Verification items for this drawing (mm, ordinates from the low corner). Give positions to 0.01 mm unless a question says otherwise; leave off trailing zeros. Write each loop counter-clockwise with the first axis right and the second up, starting at its lowest first coordinate (ties: lowest second). Pieces come first, ordered by that corner, then holes. Notation, with made-up numbers: (64.5, -33.75) -> (69.5, -33.75) arc R16 ccw to (69.5, -13.75) -> close; hole circle Ø7 at (13.5, -0.5). An arc over 180 degrees is marked (long way). Use one line per item in the form item = value. Start each with the question number.
(1) Depth check by flat-ended pin: pin 1 Ø11.5 at (x, z) = (38.1, 38.1) entering from -Y. Enter the tip coordinate at first touch or a pass-through.
(2) Scan lines: L1, parallel to Z at x = 12, y = 2.5 (3 decimals); L2, parallel to X at y = 4.5, z = 7; L3, parallel to X at y = 1.5, z = 38.1 (3 decimals). Record each from-to range of solid material in increasing order.
(3) Section check B-B, the plane x = 38.1. Record the cut outline in (y, z) (3 decimals).
(4) Section check D-D, the plane y = 4.25. Record the cut outline in (x, z) (3 decimals), plus the area to 3 significant figures.
(5) Section check C-C, the plane z = 13.5. Record the cut outline in (x, y).
(6) Section check A-A, the plane z = 38.1. Record the cut outline in (x, y) (3 decimals), plus the area to 3 significant figures.
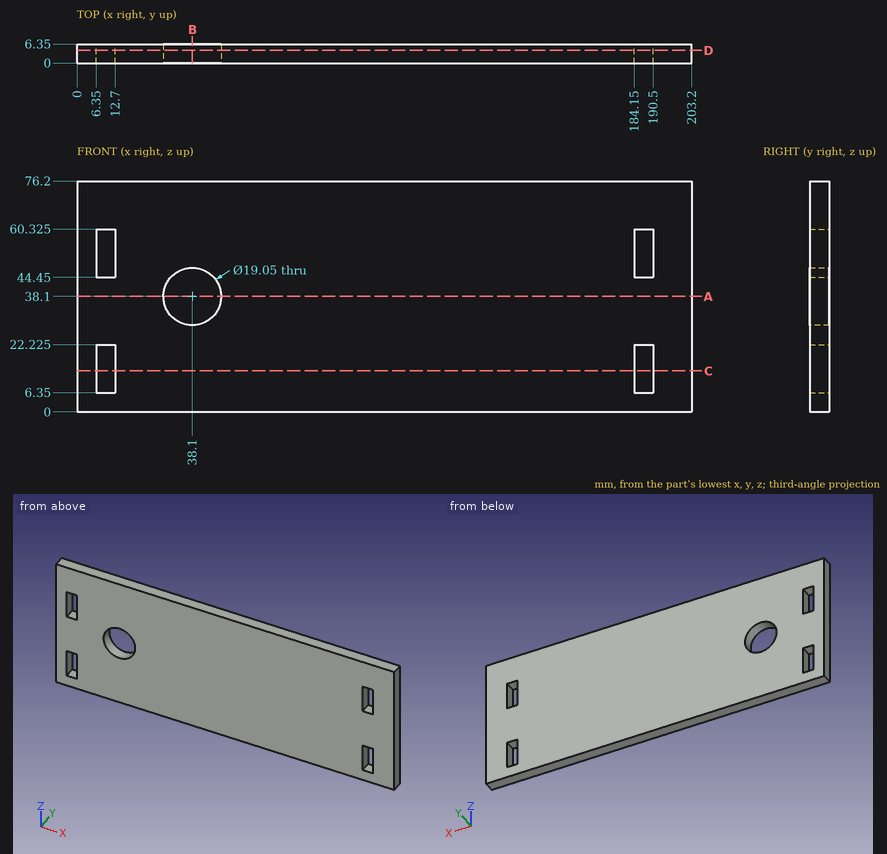
Completed:
q1.pin_1 = through
q2.L1 = 0 to 6.35, 22.225 to 44.45, 60.325 to 76.2
q2.L2 = 0 to 6.35, 12.7 to 184.15, 190.5 to 203.2
q2.L3 = 0 to 28.575, 47.625 to 203.2
q3.outline = (0, 0) -> (6.35, 0) -> (6.35, 28.575) -> (0, 28.575) -> close; (0, 47.625) -> (6.35, 47.625) -> (6.35, 76.2) -> (0, 76.2) -> close
q4.outline = (0, 0) -> (203.2, 0) -> (203.2, 76.2) -> (0, 76.2) -> close; hole (6.35, 6.35) -> (12.7, 6.35) -> (12.7, 22.225) -> (6.35, 22.225) -> close; hole (6.35, 44.45) -> (12.7, 44.45) -> (12.7, 60.325) -> (6.35, 60.325) -> close; hole circle Ø19.05 at (38.1, 38.1); hole (184.15, 6.35) -> (190.5, 6.35) -> (190.5, 22.225) -> (184.15, 22.225) -> close; hole (184.15, 44.45) -> (190.5, 44.45) -> (190.5, 60.325) -> (184.15, 60.325) -> close
q4.area = 14,800 mm²
q5.outline = (0, 0) -> (6.35, 0) -> (6.35, 6.35) -> (0, 6.35) -> close; (12.7, 0) -> (184.15, 0) -> (184.15, 6.35) -> (12.7, 6.35) -> close; (190.5, 0) -> (203.2, 0) -> (203.2, 6.35) -> (190.5, 6.35) -> close
q6.outline = (0, 0) -> (28.575, 0) -> (28.575, 6.35) -> (0, 6.35) -> close; (47.625, 0) -> (203.2, 0) -> (203.2, 6.35) -> (47.625, 6.35) -> close
q6.area = 1,170 mm²
